```python
from build123d import *

# Parameters (mm, degrees)
F0_W      = 38.10881
F0_H      = 57.533204
F1_DEPTH  = 19.05
F2_R      = 3.066051
F3_R      = 3.679261
F4_R      = 4.292472
F5_R      = 4.292472
F7_DEPTH  = 2.032
F8_R      = 4.017034
F9_DEPTH  = 2.794
F11_DEPTH = 2.286
F12_R     = 2.195821
F13_DEPTH = 3.048


with BuildPart() as f1:
    # F0 (on Front) → F1 (new body)
    with BuildSketch(Plane.XZ):
        Rectangle(F0_W, F0_H)
    extrude(amount=F1_DEPTH)

    # F2
    f2_edges = [f1.edges().sort_by_distance(p)[0] for p in [
        (19.054405, -19.05, 0),
    ]]
    fillet(f2_edges, radius=F2_R)

    # F3
    f3_edges = [f1.edges().sort_by_distance(p)[0] for p in [
        (-19.054405, -19.05, 0),
    ]]
    fillet(f3_edges, radius=F3_R)

    # F4
    f4_edges = [f1.edges().sort_by_distance(p)[0] for p in [
        (19.054405, 0, 0),
    ]]
    fillet(f4_edges, radius=F4_R)

    # F5
    f5_edges = [f1.edges().sort_by_distance(p)[0] for p in [
        (-19.054405, 0, 0),
    ]]
    fillet(f5_edges, radius=F5_R)

    # F6 (on face) → F7 (join)
    with BuildSketch(Plane.XY.offset(28.766602)):
        Polygon((-12.688468, -11.684282), (-8.879722, -11.747133), (-6.920919, -8.480087), (-8.770862, -5.150191), (-12.579608, -5.08734), (-14.538411, -8.354386), align=None)
    extrude(amount=F7_DEPTH)

    # F8 (on face) → F9 (join)
    with BuildSketch(Plane.XY.offset(28.766602)):
        with Locations((7.584764, -8.480087)):
            Circle(F8_R)
    extrude(amount=F9_DEPTH)

    # F10 (on face) → F11 (cut)
    with BuildSketch(Plane.XY.offset(30.798602)):
        Polygon((-9.831909, -10.003621), (-8.879722, -8.354386), (-9.831909, -6.70515), (-11.736282, -6.70515), (-12.688468, -8.354386), (-11.736282, -10.003621), align=None)
    extrude(amount=-F11_DEPTH, mode=Mode.SUBTRACT)

    # F12 (on face) → F13 (cut)
    with BuildSketch(Plane.XY.offset(31.560602)):
        with Locations((7.584764, -8.480087)):
            Circle(F12_R)
    extrude(amount=-F13_DEPTH, mode=Mode.SUBTRACT)


solid = f1.part
```
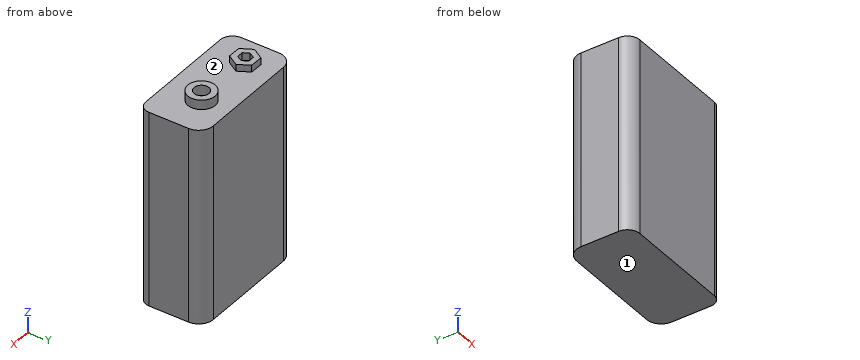
The model under review builds one solid part; all positions refer to its coordinate system, in mm. Face numbers are marked on the shaded views. A direction names the side the tool comes from. Give positions to 0.01 mm unless a question says otherwise; leave off trailing zeros. Write each loop counter-clockwise with the first axis right and the second up, starting at its lowest first coordinate (ties: lowest second). Pieces come first, ordered by that corner, then holes. Notation, with made-up numbers: (-19.75, -30) - (-4.75, -30) arc R21 cw to (-4.75, 8) - close; hole circle Ø5 at (68.5, -13). An arc over 180 degrees is marked (long way). Answer in a Markdown table with one row per item. Add a question column.
1. We need section C-C on y = -14.25. Write out the cut boundary in (x, z).
2. We need section D-D on x = 8.5. Write out the cut boundary in (y, z).
3. We need section A-A on z = 1.5. Write out the cut boundary in (x, y).
4. Insertion check: P1, Ø0.6, axis at x = -11, z = 30, coming from the -Y side; P2, Ø0.6, axis at x = -11, z = 29.5, coming from the +Y side; P3, Ø6, axis at x = -10.5, y = -14, coming from the +Z side. Each pin has a flat end and moves straight along its axis. Give the tip position at first contact, or say it passes through.
5. We need section B-B on x = -11. Write out the cut boundary in (y, z).
6. Wall thickness on line 1 along Y through (x, z) = (15, 20); line 2 along Z through (x, y) = (-3.5, -5.75); line 3 along X through (y, z) = (-15.5, -1.5): over which ranges is each line inside the solid? List them lowest first. Write a range as [from, to].
7. Tool access review of the marked faces 1 and 2: name each direction out of +Z, -Z, +X, -X, +Y, -Y from which nothing blocks a thin tool from reaching the whole face with its end or side.
Ans:
| question | item | result |
|---|---|---|
| 1 | outline | (-19.05, -28.77) - (19.05, -28.77) - (19.05, 28.77) - (-19.05, 28.77) - close |
| 2 | outline | (-19.05, -28.77) - (0, -28.77) - (0, 28.77) - (-4.57, 28.77) - (-4.57, 31.56) - (-6.48, 31.56) - (-6.48, 28.51) - (-10.48, 28.51) - (-10.48, 31.56) - (-12.39, 31.56) - (-12.39, 28.77) - (-19.05, 28.77) - close |
| 3 | outline | (-19.05, -15.37) arc R3.68 ccw to (-15.38, -19.05) - (15.99, -19.05) arc R3.07 ccw to (19.05, -15.98) - (19.05, -4.29) arc R4.29 ccw to (14.76, 0) - (-14.76, 0) arc R4.29 ccw to (-19.05, -4.29) - close |
| 4 | P1 | stops at y = -11.72 |
| 4 | P2 | stops at y = -5.11 |
| 4 | P3 | stops at z = 30.8 |
| 5 | outline | (-19.05, -28.77) - (0, -28.77) - (0, 28.77) - (-5.11, 28.77) - (-5.11, 30.8) - (-6.71, 30.8) - (-6.71, 28.51) - (-10, 28.51) - (-10, 30.8) - (-11.71, 30.8) - (-11.71, 28.77) - (-19.05, 28.77) - close |
| 6 | line 1 | y = [-19.05, -0.01] |
| 6 | line 2 | z = [-28.77, 28.77] |
| 6 | line 3 | x = [-19.05, 19.05] |
| 7 | face 1 | -Z, +X, -X, +Y, -Y |
| 7 | face 2 | +Z |
